Design review of the part built by this model. Coordinates are the model's own, in mm. A direction names the side the tool comes from. Round coordinates to 2 decimals unless told otherwise and drop trailing zeros. Order: outer loops, then holes, each group sorted by start corner. A loop starts at its lowest first (then second) coordinate and runs counter-clockwise, first axis right, second up. Notation, with made-up numbers: (-8.5, -38.75) - (16.5, -38.75) arc R37 ccw to (16.5, -0.75) - close; hole circle Ø10 at (76.5, 78.25). An arc over 180 degrees is marked (long way). Use CSV: the item, a comma, the result in double quotes. Start each with the question number.
from build123d import *

# Parameters (mm, degrees)
SKETCH1_W               = 84
SKETCH1_H               = 81
BOSS_EXTRUDE1_DEPTH     = 2
SKETCH2_R               = 1.65
BOSS_EXTRUDE2_DEPTH     = 2
MIRROR2_COPY_1_SKETCH_R = 1.65
MIRROR2_COPY_1_DEPTH    = 2
FILLET1_R               = 10
SKETCH3_R               = 1.4
CUT_EXTRUDE1_DEPTH      = 3


with BuildPart() as part:
    # Sketch1 → Boss-Extrude1 (new body)
    with BuildSketch(Plane(origin=(0, 0, 0), x_dir=(1, 0, 0), z_dir=(0, 1, 0))):
        Rectangle(SKETCH1_W, SKETCH1_H)
    extrude(amount=BOSS_EXTRUDE1_DEPTH)

    # Sketch2 → Boss-Extrude2 (add)
    with BuildSketch(Plane(origin=(0, 2, 0), x_dir=(1, 0, 0), z_dir=(0, 1, 0))):
        with BuildLine():
            Line((-42.781426662, 49.766572276), (-32.781426662, 39.879072276))
            ThreePointArc((-32.781426662, 39.879072276), (-32.733427724, 31.393926662), (-41.218573338, 31.345927724))
            Line((-41.218573338, 31.345927724), (-51.218573338, 41.233427724))
            ThreePointArc((-51.218573338, 41.233427724), (-51.266572276, 49.718573338), (-42.781426662, 49.766572276))
        make_face()
        with Locations((-47, 45.5)):
            Circle(SKETCH2_R, mode=Mode.SUBTRACT)
    boss_extrude2 = extrude(amount=-BOSS_EXTRUDE2_DEPTH)

    # Mirror1: Boss-Extrude2 across plane
    add(boss_extrude2.mirror(Plane.XY))

    # Mirror2: Boss-Extrude2 across plane
    add(boss_extrude2.mirror(Plane(origin=(0, 0, 0), x_dir=(0, 0, 1), z_dir=(1, 0, 0))))

    # Mirror2 copy 1 sketch → Mirror2 copy 1 (add)
    with BuildSketch(Plane(origin=(0, 2, 0), x_dir=(-1, 0, 0), z_dir=(0, 1, 0))):
        with BuildLine():
            Line((-42.781426662, 49.766572276), (-32.781426662, 39.879072276))
            ThreePointArc((-32.781426662, 39.879072276), (-32.733427724, 31.393926662), (-41.218573338, 31.345927724))
            Line((-41.218573338, 31.345927724), (-51.218573338, 41.233427724))
            ThreePointArc((-51.218573338, 41.233427724), (-51.266572276, 49.718573338), (-42.781426662, 49.766572276))
        make_face()
        with Locations((-47, 45.5)):
            Circle(MIRROR2_COPY_1_SKETCH_R, mode=Mode.SUBTRACT)
    extrude(amount=-MIRROR2_COPY_1_DEPTH)

    # Fillet1
    fillet1_edges = [part.edges().sort_by_distance(p)[0] for p in [
        (-42, 1, -32.118563335),
        (-33.409419303, 1, -40.5),
        (-42, 1, 32.118563335),
        (-33.409419303, 1, 40.5),
        (42, 1, -32.118563335),
        (33.409419303, 1, -40.5),
        (42, 1, 32.118563335),
        (33.409419303, 1, 40.5),
    ]]
    fillet(fillet1_edges, radius=FILLET1_R)

    # Sketch3 → Cut-Extrude1 (cut, through all)
    with BuildSketch(Plane(origin=(0, 2, 0), x_dir=(1, 0, 0), z_dir=(0, 1, 0))):
        with Locations((-29, 0)):
            Circle(SKETCH3_R)
        with Locations((29, 0)):
            Circle(SKETCH3_R)
    extrude(amount=-CUT_EXTRUDE1_DEPTH, mode=Mode.SUBTRACT)


solid = part.part
Q1. Take a section at A-A (z = 0). State the section outline as (x, y) points, plus the area to 3 significant figures.
Q2. The part is to be moulded in two halves that separate along X. For faces 4 (the cylindrical face through (42.751, 1.014, -31.745)), 5 (the cylindrical face through (33.15, 0.99, 41.27)), 6 (the cylindrical face through (-42.751, 0.986, -31.745)), 7 (the flat face through (-1, 2, 1)), say which applies: +X half, -X half, draft (parallel to the pull), parting line (faces both ways), or undercut.
Q3. Tool access review of faces 1 (the flat face through (-48.05, 1.01, 38.1)), 2 (the flat face through (39.6, 1.01, 46.62)), 3 (the flat face through (39.6, 1.01, -46.62)): name each direction out of +Z, -Z, +X, -X, +Y, -Y from which nothing blocks a thin tool from reaching the whole face with its end or side.
Q4. Take a section at D-D (x = -11). State the section outline as (y, z) points, plus the area to 3 significant figures.
Q5. Take a section at C-C (z = -45.5). State the section outline as (x, y) points.
Q6. For L1, parallel to X at y = 0.85, z = 0; L2, parallel to Z at x = 47, y = 0.95; L3, parallel to X at y = 1.45, z = -45.5, list the stretches that pass through material, from the lowest coordinate up. Write a range as [from, to].
Q7. Take a section at B-B (y = 1.4). Give the number of separate pieces and of enclosed holes in the cut face, plus the area to 3 significant figures.
Q8. Clearance check with flat-ended pins moving along their axes: pin 1 (1 mm diameter, centred on y = 0.5, z = 34.5, fed in from -X); pin 2 (0.6 mm diameter, centred on y = 1, z = 10.5, fed in from +X); pin 3 (1 mm diameter, centred on y = 0.5, z = -13.5, fed in from -X). State where each tip first meets the part, or that it passes through.
Findings below:
1,outline,"(-42, 0) - (-30.4, 0) - (-30.4, 2) - (-42, 2) - close; (-27.6, 0) - (27.6, 0) - (27.6, 2) - (-27.6, 2) - close; (30.4, 0) - (42, 0) - (42, 2) - (30.4, 2) - close"
1,area,"157 mm^2"
2,face 4,"+X half"
2,face 5,"undercut"
2,face 6,"-X half"
2,face 7,"draft"
3,face 1,"-X, +Y, -Y"
3,face 2,"+Z, +Y, -Y"
3,face 3,"-Z, +Y, -Y"
4,outline,"(0, -40.5) - (2, -40.5) - (2, 40.5) - (0, 40.5) - close"
4,area,"162 mm^2"
5,outline,"(-53, 0) - (-48.65, 0) - (-48.65, 2) - (-53, 2) - close; (-45.35, 0) - (-38.47, 0) - (-38.47, 2) - (-45.35, 2) - close; (38.47, 0) - (45.35, 0) - (45.35, 2) - (38.47, 2) - close; (48.65, 0) - (53, 0) - (53, 2) - (48.65, 2) - close"
6,L1,"x = [-42, -30.4], [-27.6, 27.6], [30.4, 42]"
6,L2,"z = [-51.5, -47.15], [-43.85, -37.06], [37.06, 43.85], [47.15, 51.5]"
6,L3,"x = [-53, -48.65], [-45.35, -38.47], [38.47, 45.35], [48.65, 53]"
7,separate pieces,"1"
7,enclosed holes,"6"
7,area,"7,480 mm^2"
8,pin 1,"stops at x = -44.91"
8,pin 2,"stops at x = 42"
8,pin 3,"stops at x = -42"
